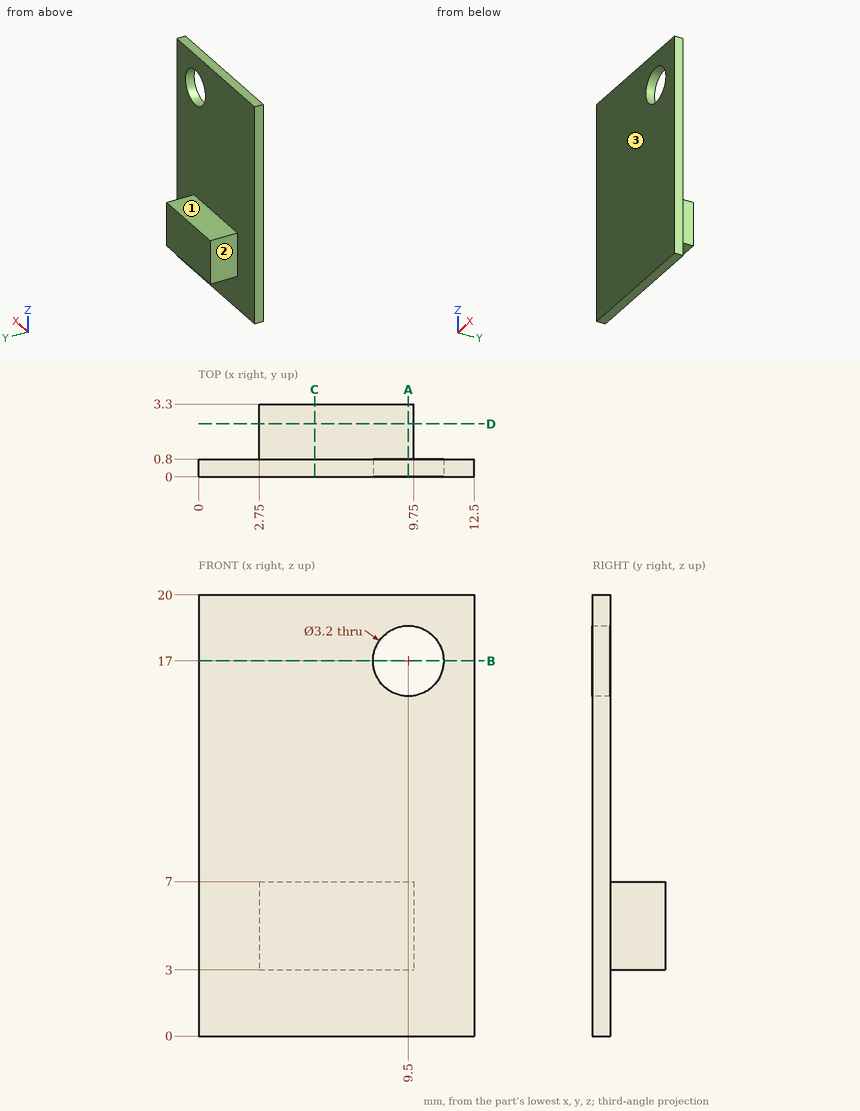
Answer from the drawing. Dimensions are ordinates in mm from the lowest x, y and z of the part. A direction names the side the tool comes from. Coordinates: 2 decimals unless noted, no trailing zeros. Order: outer loops, then holes, each group sorted by start corner. A loop starts at its lowest first (then second) coordinate and runs counter-clockwise, first axis right, second up. Notation, with made-up numbers: (32.25, -25.5) - (37.25, -25.5) arc R20 ccw to (37.25, 2.5) - close; hole circle Ø5 at (77.25, -14). An arc over 180 degrees is marked (long way). Answer as a JSON object with one key per item and string values. Group by question number.
Item 1: Section C-C (x = 5.25) is taken. Give the vertices of the cut face in (y, z), plus the area to 3 significant figures.
Item 2: Section B-B (z = 17) is taken. Give the vertices of the cut face in (x, y).
Item 3: Flat-ended cylindrical pins translate along their axes: P1, Ø0.8, axis at x = 5.5, y = 2, coming from the -Z side; P2, Ø1, axis at y = 1, z = 13, coming from the -X side; P3, Ø0.8, axis at y = 2, z = 4.5, coming from the -X side; P4, Ø1.5, axis at x = 1.5, z = 9.5, coming from the +Y side. Find the tip coordinate at first contact, or state that the pin passes through.
Item 4: Section A-A (x = 9.5) is taken. Give the vertices of the cut face in (y, z), plus the area to 3 significant figures.
Item 5: Consider probe 1 along X at (y, z) = (0.5, 17); probe 2 along Z at (x, y) = (6.25, 0.95); probe 3 along Y at (x, z) = (4.5, 9.5). Determine where each line is inside the solid, lowest interval first. Write a range as from..to.
Item 6: Section D-D (y = 2.4) is taken. Give the vertices of the cut face in (x, z).
Item 7: A tool of negligible diameter and unlimited length cuts with its end or side. For the marked faces 1, 2 and 3, from which of +Z, -Z, +X, -X, +Y, -Y can it reach the whole face along a straight path? Write none if from no direction.
Results are:
{
 "1": {"outline": "(0, 0) - (0.8, 0) - (0.8, 3) - (3.3, 3) - (3.3, 7) - (0.8, 7) - (0.8, 20) - (0, 20) - close", "area": "26.0 mm^2"},
 "2": {"outline": "(0, 0) - (7.9, 0) - (7.9, 0.8) - (0, 0.8) - close; (11.1, 0) - (12.5, 0) - (12.5, 0.8) - (11.1, 0.8) - close"},
 "3": {"P1": "stops at z = 3", "P2": "stops at x = 0", "P3": "stops at x = 2.75", "P4": "stops at y = 0.8"},
 "4": {"outline": "(0, 0) - (0.8, 0) - (0.8, 3) - (3.3, 3) - (3.3, 7) - (0.8, 7) - (0.8, 15.4) - (0, 15.4) - close; (0, 18.6) - (0.8, 18.6) - (0.8, 20) - (0, 20) - close", "area": "23.4 mm^2"},
 "5": {"probe 1": "x = 0..7.9, 11.1..12.5", "probe 2": "z = 3..7", "probe 3": "y = 0..0.8"},
 "6": {"outline": "(2.75, 3) - (9.75, 3) - (9.75, 7) - (2.75, 7) - close"},
 "7": {"face 1": "+Z, +X, -X, +Y", "face 2": "+Z, -Z, -X, +Y", "face 3": "+Z, -Z, +X, -X, -Y"}
}
